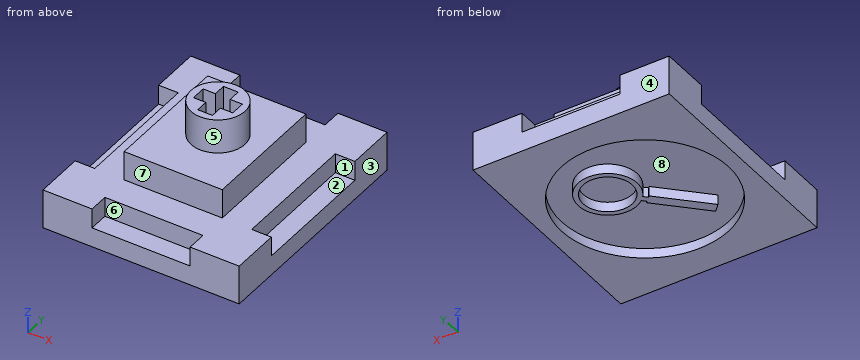
Autodesk Fusion 360 part; units mm, degrees
sketch "スケッチ1" plane through (0, 0, 0) normal (0, 0, 1) x (1, 0, 0)
  line L0 (0, 0) -> (20, 0)
  line L1 (20, 0) -> (20, 23)
  line L2 (20, 23) -> (0, 23)
  line L3 (0, 23) -> (0, 0)
  dimension "d1" = 20
  dimension "d2" = 23
extrude "押し出し1" add sketch "スケッチ1" along normal blind 2
sketch "スケッチ2" plane through (0, 0, 2) normal (0, 0, 1) x (-1, 0, 0)
  line L0 (0, -23) -> (0, 0)
  line L1 (0, 0) -> (-20, 0)
  line L2 (-20, 0) -> (-20, -23)
  line L3 (-20, -23) -> (0, -23)
  line L4 (0, -23) -> (-5, -23)
  line L5 (-5, -23) -> (-5, -18)
  line L6 (-5, -18) -> (0, -18)
  line L7 (0, -18) -> (0, -23)
  line L8 (-20, -23) -> (-15, -23)
  line L9 (-15, -23) -> (-15, -18)
  line L10 (-15, -18) -> (-20, -18)
  line L11 (-20, -18) -> (-20, -23)
  line L12 (0, 0) -> (-5, 0)
  line L13 (-5, 0) -> (-5, -5)
  line L14 (-5, -5) -> (0, -5)
  line L15 (0, -5) -> (0, 0)
  line L16 (-20, 0) -> (-15, 0)
  line L17 (-15, 0) -> (-15, -5)
  line L18 (-15, -5) -> (-20, -5)
  line L19 (-20, -5) -> (-20, 0)
  line L20 (-2, -21) -> (-18, -21)
  line L21 (-18, -21) -> (-18, -2)
  line L22 (-18, -2) -> (-2, -2)
  line L23 (-2, -2) -> (-2, -21)
  dimension "d5" = 5
  dimension "d6" = 5
  dimension "d7" = 5
  dimension "d8" = 5
  dimension "d9" = 5
  dimension "d10" = 5
  dimension "d11" = 5
  dimension "d12" = 5
extrude "押し出し2" add sketch "スケッチ2" along normal blind 2 contours L0 L3 L4 L5 L6 L7 L20 L23 | L0 L1 L12 L13 L14 L15 L22 L23 | L5 L6 L20 L23 | L5 L6 L9 L10 L13 L14 L17 L18 L20 L21 L22 L23 | L2 L3 L8 L9 L10 L11 L20 L21 | L13 L14 L22 L23 | L9 L10 L20 L21 | L1 L2 L16 L17 L18 L19 L21 L22 | L17 L18 L21 L22
sketch "スケッチ3" plane through (0, 0, 4) normal (0, 0, 1) x (-1, 0, 0)
  line L0 (-18, -18) -> (-20, -18)
  line L1 (-20, -18) -> (-20, -23)
  line L2 (-20, -23) -> (-15, -23)
  line L3 (-15, -23) -> (-15, -21)
  line L4 (-15, -21) -> (-5, -21)
  line L5 (-5, -21) -> (-5, -23)
  line L6 (-5, -23) -> (0, -23)
  line L7 (0, -23) -> (0, -18)
  line L8 (0, -18) -> (-2, -18)
  line L9 (-2, -18) -> (-2, -5)
  line L10 (-2, -5) -> (0, -5)
  line L11 (0, -5) -> (0, 0)
  line L12 (0, 0) -> (-5, 0)
  line L13 (-5, 0) -> (-5, -2)
  line L14 (-5, -2) -> (-15, -2)
  line L15 (-15, -2) -> (-15, 0)
  line L16 (-15, 0) -> (-20, 0)
  line L17 (-20, 0) -> (-20, -5)
  line L18 (-20, -5) -> (-18, -5)
  line L19 (-18, -5) -> (-18, -18)
  line L20 (-5, -18) -> (-15, -18)
  line L21 (-15, -18) -> (-15, -5)
  line L22 (-15, -5) -> (-5, -5)
  line L23 (-5, -5) -> (-5, -18)
extrude "押し出し3" add sketch "スケッチ3" along normal blind 3 contours L20 L21 L22 L23
sketch "スケッチ4" plane through (0, 0, 7) normal (0, 0, 1) x (-1, 0, 0)
  line L0 (-5, -5) -> (-15, -5)
  line L1 (-15, -5) -> (-15, -18)
  line L2 (-15, -18) -> (-5, -18)
  line L3 (-5, -18) -> (-5, -5)
  line L4 (-9.55, -13.5) -> (-11.05, -13.5)
  line L5 (-11.05, -13.5) -> (-11.05, -9.5)
  line L6 (-11.05, -9.5) -> (-9.55, -9.5)
  line L7 (-9.55, -9.5) -> (-9.55, -13.5)
  line L8 (-8.3, -12.25) -> (-12.3, -12.25)
  line L9 (-12.3, -12.25) -> (-12.3, -10.75)
  line L10 (-12.3, -10.75) -> (-8.3, -10.75)
  line L11 (-8.3, -10.75) -> (-8.3, -12.25)
  circle A0 centre (-10.3, -11.5) radius 2.75
  dimension "d17" = 13
  dimension "d18" = 1.5
  dimension "d19" = 4
  dimension "d20" = 4
  dimension "d21" = 1.5
  dimension "d22" = 5.5
extrude "押し出し4" add sketch "スケッチ4" along normal blind 3.5 contours A0
sketch "スケッチ5" plane through (0, 0, 0) normal (0, 0, -1) x (1, 0, 0)
  line L0 (0, 0) -> (0, -23)
  line L1 (0, -23) -> (20, -23)
  line L2 (20, -23) -> (20, 0)
  line L3 (20, 0) -> (0, 0)
  circle A0 centre (10, -11.5) radius 8.5
  circle A1 centre (12.3008, -13.7867) radius 3
  circle A2 centre (12.3008, -13.7867) radius 2.5
  line L4 (5.2298, -7.4227) -> (5.9369, -6.7156)
  line L5 (5.9369, -6.7156) -> (10.1795, -10.9583)
  line L6 (10.1795, -10.9583) -> (9.4724, -11.6654)
  line L7 (9.4724, -11.6654) -> (5.2298, -7.4227)
  line L8 (9.978, -11.8882) -> (10.4023, -11.4639)
  line L9 (9.6138, -11.524) -> (9.978, -11.8882)
  line L10 (10.4023, -11.4639) -> (10.0381, -11.0997)
  line L11 (10.0381, -11.0997) -> (9.6138, -11.524)
extrude "押し出し5" cut sketch "スケッチ5" against normal blind 1 contours A0 | A2
Here's how the part is built. I have some questions about the finished solid (model axes, mm). Face numbers are marked on the shaded views. A direction names the side the tool comes from. Round coordinates to 2 decimals unless told otherwise and drop trailing zeros. Order: outer loops, then holes, each group sorted by start corner. A loop starts at its lowest first (then second) coordinate and runs counter-clockwise, first axis right, second up. Notation, with made-up numbers: (45, 62) -> (66, 62) arc R16 ccw to (66, 68) -> close; hole circle Ø3 at (-16, 52.25). An arc over 180 degrees is marked (long way). Return JSON: item names as keys, results as strings.
Q1. If we section it at D-D on y = 3.75: List the corners of the cut face in (x, z) for me, plus the area to 3 significant figures.
Filled sheet:
{"outline": "(0, 0) -> (6.51, 0) -> (6.51, 1) -> (13.49, 1) -> (13.49, 0) -> (20, 0) -> (20, 4) -> (0, 4) -> close", "area": "73.0 mm^2"}
Q2. If we section it at C-C on z = 3: List the corners of the cut face in (x, y) for me, plus the area to 3 significant figures.
Filled sheet:
{"outline": "(0, 0) -> (5, 0) -> (5, 2) -> (15, 2) -> (15, 0) -> (20, 0) -> (20, 5) -> (18, 5) -> (18, 18) -> (20, 18) -> (20, 23) -> (15, 23) -> (15, 21) -> (5, 21) -> (5, 23) -> (0, 23) -> (0, 18) -> (2, 18) -> (2, 5) -> (0, 5) -> close", "area": "368 mm^2"}
Q3. I need wall thicknesses on line 1 along X through (y, z) = (1.5, 3.5); line 2 along Z through (x, y) = (14.25, 19.5); line 3 along Z through (x, y) = (13, 5.75). Which ranges of each line are inside material? Lowest first, please. Write a range as from..to.
Filled sheet:
{"line 1": "x = 0..5, 15..20", "line 2": "z = 0..4", "line 3": "z = 1..7"}
Q4. If we section it at B-B on z = 7.75: List the corners of the cut face in (x, y) for me, plus the area to 3 significant figures.
Filled sheet:
{"outline": "circle Ø5.5 at (10.3, 11.5); hole (8.3, 10.75) -> (9.55, 10.75) -> (9.55, 9.5) -> (11.05, 9.5) -> (11.05, 10.75) -> (12.3, 10.75) -> (12.3, 12.25) -> (11.05, 12.25) -> (11.05, 13.5) -> (9.55, 13.5) -> (9.55, 12.25) -> (8.3, 12.25) -> close", "area": "14.0 mm^2"}
Q5. If we section it at A-A on x = 2.5: List the corners of the cut face in (y, z) for me, plus the area to 3 significant figures.
Filled sheet:
{"outline": "(0, 0) -> (7.5, 0) -> (7.5, 1) -> (15.5, 1) -> (15.5, 0) -> (23, 0) -> (23, 4) -> (0, 4) -> close", "area": "84.0 mm^2"}
Q6. If we mould it in two halves opening along Y, with no side actions, what happens to the marked faces 1, 2, 3 and 4? For each: released by +Y, released by -Y, zero draft, split by the parting line, or undercut.
Filled sheet:
{"face 1": "undercut", "face 2": "undercut", "face 3": "zero draft", "face 4": "released by +Y"}
Q7. For pin 1 Ø2.5 at (y, z) = (13, 6) entering from +X; pin 2 Ø2 at (x, z) = (7.5, 6) entering from -Y; pin 3 Ø0.9 at (x, z) = (9, 6) entering from +Y, each with a flat end and sliding along its axis, tell me the tip position at first contact or that it passes through.
Filled sheet:
{"pin 1": "stops at x = 15", "pin 2": "stops at y = 5", "pin 3": "stops at y = 18"}
Q8. Which directions (+Z, -Z, +X, -X, +Y, -Y) give clear straight access to the entire face, cutting with the end or side of a thin tool? Please do the marked faces 5, 6, 7 and 8.
Filled sheet:
{"face 5": "+Z", "face 6": "+Z, -Y", "face 7": "+Z, +X, -X, -Y", "face 8": "-Z"}
